Model file for the job. Use its own axes, mm. Give positions to 0.01 mm unless a question says otherwise; leave off trailing zeros. Write each loop counter-clockwise with the first axis right and the second up, starting at its lowest first coordinate (ties: lowest second). Pieces come first, ordered by that corner, then holes. Notation, with made-up numbers: (25.5, -19.5) - (38.5, -19.5) arc R24 cw to (38.5, -1.5) - close; hole circle Ø3 at (-35, -1.75). An arc over 180 degrees is marked (long way). Use CSV: the item, a comma, the result in double quotes.
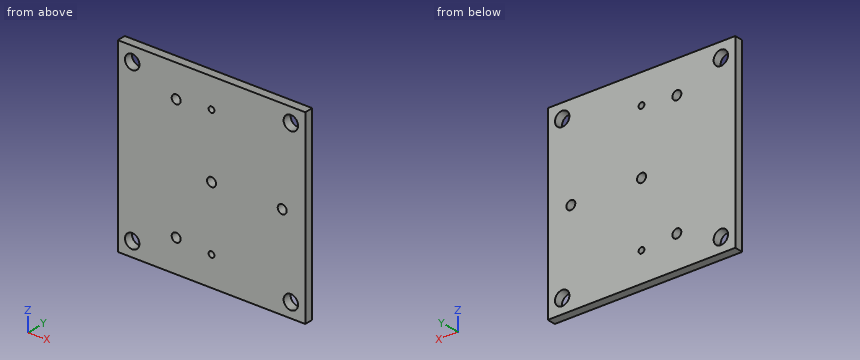
from build123d import *

# Parameters (mm, degrees)
SKETCH_8_R          = 58
SKETCH_8_R_2        = 3
EXTRUDE_5_DEPTH     = 6
SKETCH_9_R          = 2
EXTRUDE_6_DEPTH     = 12
EXTRUDE_START       = -6
SKETCH_10_W         = 130
SKETCH_10_H         = 130
SKETCH_10_R         = 5
SKETCH_10_R_2       = 58
EXTRUDE_8_DEPTH     = 6
CUT_EXTRUDE_START   = -30
SKETCH_12_R         = 2
CUT_EXTRUDE_1_DEPTH = 30
SKETCH_13_R         = 2
CUT_EXTRUDE_2_DEPTH = 30
SKETCH_14_R         = 3.1
CUT_EXTRUDE_3_DEPTH = 6
SKETCH_15_R         = 3.1
CUT_EXTRUDE_4_DEPTH = 6


with BuildPart() as part:
    # 草图8 → 凸台-拉伸5 (new body)
    with BuildSketch(Plane.XZ.offset(-1803)):
        with Locations(Location((2814.779756067, -929.5, 0), (0, 0, 270))):
            Circle(SKETCH_8_R)
        with Locations(Location((2814.779756067, -929.5, 0), (0, 0, 270))):
            Circle(SKETCH_8_R_2, mode=Mode.SUBTRACT)
    extrude(amount=EXTRUDE_5_DEPTH)

    # 草图9 → 凸台-拉伸6 (add)
    with BuildSketch(Plane.XZ.offset(-1797)):
        with Locations(Location((2814.779756067, -885.05, 0), (0, 0, 270))):
            Circle(SKETCH_9_R)
        with Locations(Location((2814.779756067, -973.95, 0), (0, 0, 270))):
            Circle(SKETCH_9_R)
    extrude(amount=-EXTRUDE_6_DEPTH)

    # 草图10 → 凸台-拉伸8 (add)
    with BuildSketch(Plane.XZ.offset(-1797).offset(EXTRUDE_START)):
        with Locations((2814.779756067, -929.5)):
            Rectangle(SKETCH_10_W, SKETCH_10_H)
        with Locations(Location((2869.779756067, -984.5, 0), (0, 0, 270))):
            Circle(SKETCH_10_R, mode=Mode.SUBTRACT)
        with Locations(Location((2759.779756067, -984.5, 0), (0, 0, 270))):
            Circle(SKETCH_10_R, mode=Mode.SUBTRACT)
        with Locations(Location((2759.779756067, -874.5, 0), (0, 0, 270))):
            Circle(SKETCH_10_R, mode=Mode.SUBTRACT)
        with Locations(Location((2869.779756067, -874.5, 0), (0, 0, 270))):
            Circle(SKETCH_10_R, mode=Mode.SUBTRACT)
        with Locations((2814.779756067, -929.5)):
            Circle(SKETCH_10_R_2, mode=Mode.SUBTRACT)
    extrude(amount=EXTRUDE_8_DEPTH)

    # 草图12 → 切除-拉伸1 (cut)
    with BuildSketch(Plane(origin=(0, 1809, 0), x_dir=(1, 0, 0), z_dir=(0, 1, 0)).offset(CUT_EXTRUDE_START)):
        with Locations(Location((2814.779756067, 973.95, 0), (0, 0, 90))):
            Circle(SKETCH_12_R)
    extrude(amount=CUT_EXTRUDE_1_DEPTH, mode=Mode.SUBTRACT)

    # 草图13 → 切除-拉伸2 (cut)
    with BuildSketch(Plane(origin=(0, 1809, 0), x_dir=(1, 0, 0), z_dir=(0, 1, 0)).offset(CUT_EXTRUDE_START)):
        with Locations(Location((2814.779756067, 885.05, 0), (0, 0, 90))):
            Circle(SKETCH_13_R)
    extrude(amount=CUT_EXTRUDE_2_DEPTH, mode=Mode.SUBTRACT)

    # 草图14 → 切除-拉伸3 (cut)
    with BuildSketch(Plane(origin=(0, 1803, 0), x_dir=(1, 0, 0), z_dir=(0, 1, 0))):
        with Locations(Location((2814.779756067, 929.5, 0), (0, 0, 270))):
            Circle(SKETCH_14_R)
    extrude(amount=-CUT_EXTRUDE_3_DEPTH, mode=Mode.SUBTRACT)

    # 草图15 → 切除-拉伸4 (cut)
    with BuildSketch(Plane(origin=(0, 1803, 0), x_dir=(1, 0, 0), z_dir=(0, 1, 0))):
        with Locations(Location((2863.779756067, 929.5, 0), (0, 0, 270))):
            Circle(SKETCH_15_R)
        with Locations(Location((2790.279756067, 887.064755215, 0), (0, 0, 270))):
            Circle(SKETCH_15_R)
        with Locations(Location((2790.279756067, 971.935244785, 0), (0, 0, 270))):
            Circle(SKETCH_15_R)
    extrude(amount=-CUT_EXTRUDE_4_DEPTH, mode=Mode.SUBTRACT)


solid = part.part
(1) Saw through at A-A, the plane z = -929.5. List the corners of the cut face in (x, y), then the cut area to 3 significant figures.
Checked values:
outline,"(2749.78, 1797) - (2811.68, 1797) - (2811.68, 1803) - (2749.78, 1803) - close; (2817.88, 1797) - (2860.68, 1797) - (2860.68, 1803) - (2817.88, 1803) - close; (2866.88, 1797) - (2879.78, 1797) - (2879.78, 1803) - (2866.88, 1803) - close"
area,"706 mm^2"
(2) Wall check: probe 1 along X at (y, z) = (1801.3, -874.5); probe 2 along X at (y, z) = (1799.95, -980.5); probe 3 along Z at (x, y) = (2762, 1801). Give the ranges that are in metal, low to high. Write a range as [from, to].
Checked values:
probe 1,"x = [2749.78, 2754.78], [2764.78, 2864.78], [2874.78, 2879.78]"
probe 2,"x = [2749.78, 2756.78], [2762.78, 2866.78], [2872.78, 2879.78]"
probe 3,"z = [-994.5, -988.98], [-980.02, -878.98], [-870.02, -864.5]"
(3) Saw through at B-B, the plane y = 1799.75. Count the separate pieces of the cut face and the enclosed holes in it, then the cut area to 3 significant figures.
Checked values:
separate pieces,"1"
enclosed holes,"10"
area,"16,400 mm^2"
(4) Saw through at C-C, the plane z = -874.5. List the corners of the cut face in (x, y), then the cut area to 3 significant figures.
Checked values:
outline,"(2749.78, 1797) - (2754.78, 1797) - (2754.78, 1803) - (2749.78, 1803) - close; (2764.78, 1797) - (2864.78, 1797) - (2864.78, 1803) - (2764.78, 1803) - close; (2874.78, 1797) - (2879.78, 1797) - (2879.78, 1803) - (2874.78, 1803) - close"
area,"660 mm^2"
